Input: part model. Units: mm. Frame: model coordinates. A direction names the side the tool comes from. Give positions to 0.01 mm unless a question says otherwise; leave off trailing zeros. Loops run counter-clockwise (first coordinate to the right, second up) from the corner with the lowest first, then second, coordinate; pieces in that order, holes last. Notation, with made-up numbers: (41.5, -36) - (97.5, -36) arc R14 ccw to (97.5, -9) - close; hole circle Ø10 at (37.5, 48.25). An arc over 180 degrees is marked (long way). Answer as a JSON object with one key per item and string values. Group by question number.
(1) Mould query, pull axis Y, two halves, no side actions, for faces 1 (the flat face through (-29, -41.222, -12)), 2 (the flat face through (-27.9, -34.7, -7.2)), 3 (the cylindrical face through (-56.978, -10.627, -8.218)), 4 (the flat face through (-51, -8, 1.765)). Classes: +Y half, -Y half, draft (parallel to the pull), parting line (faces both ways), or undercut.
(2) Section query D-D (y = -31.5). Return loops of the section in (x, z).
(3) Pin query (flat end, axial travel): P1, Ø9, axis at x = -21.5, y = -17.5, coming from the -Z side; P2, Ø1.8, axis at x = -3, y = -12.5, coming from the +Z side; P3, Ø1, axis at x = -61, y = -22, coming from the +Z side. Return the tip coordinate at first contact, or that it passes through.
(4) Section query C-C (x = -14.5). Return loops of the section in (y, z).
(5) Material intervals for L1, parallel to Y at x = -25.5, z = -1; L2, parallel to X at y = -37.5, z = -5.5; L3, parallel to Z at x = -56, y = -10, sorted ascending.
(6) Section query A-A (z = -21.5). Return loops of the section in (x, y).
(7) Section query B-B (y = -24). Return loops of the section in (x, z).
(8) Access query for faces 5 (the flat face through (-32.024, -32, -7)), 6 (the flat face through (-61, -24, 1.6)), 7 (the flat face through (-30, -39.222, -20)), 8 (the cylindrical face through (-2.82, -13.2, -27.97)). Directions: +Z, -Z, +X, -X, +Y, -Y. A direction counts if a zero-diameter tool reaches every point of the face in a straight line with its end or side. Return the directions, or none.
```python
from build123d import *

# Parameters (mm, degrees)
SKETCH_2_W           = 65.2997206
SKETCH_2_H           = 34.311658624
SKETCH_2_R           = 1.00000254
SKETCH_2_R_2         = 0.922218434
SKETCH_2_R_3         = 1.5
EXTRUDE_2_DEPTH      = 4.5
SKETCH_3_R           = 1.5
CUT_EXTRUDE_2_DEPTH  = 2.5
SKETCH_5_W           = 65.2997206
SKETCH_5_H           = 34.311658624
SKETCH_5_W_2         = 61.2997206
SKETCH_5_H_2         = 30.311658624
EXTRUDE_3_DEPTH      = 15.5
EXTRUDE_3_DEPTH_BACK = 16
SKETCH_7_W           = 8.214112973
SKETCH_7_H           = 3.795011114
CUT_EXTRUDE_4_DEPTH  = 3
SKETCH_8_W           = 4
SKETCH_8_H           = 9.575559499
CUT_EXTRUDE_5_DEPTH  = 3
SKETCH_9_W           = 9.326303795
SKETCH_9_H           = 4.202278939
CUT_EXTRUDE_6_DEPTH  = 3
SKETCH_10_W          = 65.2997206
SKETCH_10_H          = 34.311658624
SKETCH_10_R          = 1
EXTRUDE_4_DEPTH      = 4


with BuildPart() as part:
    # 草图2 → 凸台-拉伸2 (new body)
    with BuildSketch(Plane(origin=(0, 0, -6), x_dir=(-1, 0, 0), z_dir=(0, 0, -1))):
        with Locations((29.273558547, -24.066548133)):
            Rectangle(SKETCH_2_W, SKETCH_2_H)
        with Locations((1.016002032, -11.24978156)):
            Circle(SKETCH_2_R, mode=Mode.SUBTRACT)
        with Locations((0.889001778, -36.83007366)):
            Circle(SKETCH_2_R, mode=Mode.SUBTRACT)
        with Locations((57.658115316, -36.64983236)):
            Circle(SKETCH_2_R, mode=Mode.SUBTRACT)
        with Locations((57.658115316, -11.24978156)):
            Circle(SKETCH_2_R_2, mode=Mode.SUBTRACT)
        with Locations((29.273558547, -32.316548133)):
            Circle(SKETCH_2_R_3, mode=Mode.SUBTRACT)
        with BuildLine():
            Line((27.785407033, -15.816548133), (27.785407033, -13.183619987))
            ThreePointArc((27.785407033, -13.183619987), (29.273558547, -11.695468472), (30.761710061, -13.183619987))
            Line((30.761710061, -13.183619987), (30.761710061, -15.816548133))
            ThreePointArc((30.761710061, -15.816548133), (29.273558547, -17.304699647), (27.785407033, -15.816548133))
        make_face(mode=Mode.SUBTRACT)
    extrude(amount=EXTRUDE_2_DEPTH)

    # 草图3 → 切除-拉伸2 (cut)
    with BuildSketch(Plane(origin=(0, 0, -6), x_dir=(-1, 0, 0), z_dir=(0, 0, -1))):
        Polygon((29.273558547, -18.991974614), (32.023558547, -17.404261373), (32.023558547, -14.920341582), (32.023558547, -14.228834893), (32.023558547, -11.744915102), (29.273558547, -10.157201862), (26.523558547, -11.744915102), (26.523558547, -14.228834893), (26.523558547, -14.920341582), (26.523558547, -17.404261373), align=None)
        with BuildLine():
            ThreePointArc((30.761710061, -15.816548133), (29.273558547, -17.304699647), (27.785407033, -15.816548133))
            Line((27.785407033, -15.816548133), (27.785407033, -13.183619987))
            ThreePointArc((27.785407033, -13.183619987), (29.273558547, -11.695468472), (30.761710061, -13.183619987))
            Line((30.761710061, -13.183619987), (30.761710061, -15.816548133))
        make_face(mode=Mode.SUBTRACT)
        Polygon((26.523558547, -30.728834893), (26.523558547, -33.904261373), (29.273558547, -35.491974614), (32.023558547, -33.904261373), (32.023558547, -30.728834893), (29.273558547, -29.141121653), align=None)
        with Locations((29.273558547, -32.316548133)):
            Circle(SKETCH_3_R, mode=Mode.SUBTRACT)
    extrude(amount=CUT_EXTRUDE_2_DEPTH, mode=Mode.SUBTRACT)

    # 草图5 → 凸台-拉伸3 (add, two sides)
    with BuildSketch(Plane(origin=(0, 0, -10.5), x_dir=(-1, 0, 0), z_dir=(0, 0, -1))) as extrude_3_sk:
        with Locations((29.273558547, -24.066548133)):
            Rectangle(SKETCH_5_W, SKETCH_5_H)
        with Locations((29.273558547, -24.066548133)):
            Rectangle(SKETCH_5_W_2, SKETCH_5_H_2, mode=Mode.SUBTRACT)
    extrude(amount=EXTRUDE_3_DEPTH)
    extrude(extrude_3_sk.sketch, amount=-EXTRUDE_3_DEPTH_BACK)

    # 草图7 → 切除-拉伸4 (cut)
    with BuildSketch(Plane(origin=(0, -6.910718821, 0), x_dir=(1, 0, 0), z_dir=(0, 1, 0))):
        with Locations((-50.955145133, -3.662545243)):
            Rectangle(SKETCH_7_W, SKETCH_7_H)
    extrude(amount=-CUT_EXTRUDE_4_DEPTH, mode=Mode.SUBTRACT)

    # 草图8 → 切除-拉伸5 (cut)
    with BuildSketch(Plane.ZY.offset(61.923418847)):
        with Locations((3.6000508, -23.483057223)):
            Rectangle(SKETCH_8_W, SKETCH_8_H)
    extrude(amount=-CUT_EXTRUDE_5_DEPTH, mode=Mode.SUBTRACT)

    # 草图9 → 切除-拉伸6 (cut)
    with BuildSketch(Plane.XZ.offset(41.222377445)):
        with Locations((-44.464129124, 3.49891133)):
            Rectangle(SKETCH_9_W, SKETCH_9_H)
    extrude(amount=-CUT_EXTRUDE_6_DEPTH, mode=Mode.SUBTRACT)

    # 草图10 → 凸台-拉伸4 (add)
    with BuildSketch(Plane(origin=(0, 0, -26), x_dir=(-1, 0, 0), z_dir=(0, 0, -1))):
        with Locations((29.273558547, -24.066548133)):
            Rectangle(SKETCH_10_W, SKETCH_10_H)
        Polygon((-1.376301753, -14.910718821), (-1.376301753, -8.910718821), (4.623698247, -8.910718821), (53.923418847, -8.910718821), (59.923418847, -8.910718821), (59.923418847, -14.910718821), (59.923418847, -33.222377445), (59.923418847, -39.222377445), (53.923418847, -39.222377445), (4.623698247, -39.222377445), (-1.376301753, -39.222377445), (-1.376301753, -33.222377445), align=None, mode=Mode.SUBTRACT)
        with BuildLine():
            Line((4.623698247, -8.910718821), (-1.376301753, -8.910718821))
            Line((-1.376301753, -8.910718821), (-1.376301753, -14.910718821))
            ThreePointArc((-1.376301753, -14.910718821), (2.866338935, -13.153359509), (4.623698247, -8.910718821))
        make_face()
        with Locations((1.016002032, -11.24978156)):
            Circle(SKETCH_10_R, mode=Mode.SUBTRACT)
        with BuildLine():
            ThreePointArc((4.623698247, -39.222377445), (2.866338935, -34.979736758), (-1.376301753, -33.222377445))
            Line((-1.376301753, -33.222377445), (-1.376301753, -39.222377445))
            Line((-1.376301753, -39.222377445), (4.623698247, -39.222377445))
        make_face()
        with Locations((1.016002032, -36.883314707)):
            Circle(SKETCH_10_R, mode=Mode.SUBTRACT)
        with BuildLine():
            Line((59.923418847, -39.222377445), (59.923418847, -33.222377445))
            ThreePointArc((59.923418847, -33.222377445), (55.68077816, -34.979736758), (53.923418847, -39.222377445))
            Line((53.923418847, -39.222377445), (59.923418847, -39.222377445))
        make_face()
        with Locations((57.658115316, -36.883314707)):
            Circle(SKETCH_10_R, mode=Mode.SUBTRACT)
        with BuildLine():
            Line((59.923418847, -8.910718821), (53.923418847, -8.910718821))
            ThreePointArc((53.923418847, -8.910718821), (55.68077816, -13.153359509), (59.923418847, -14.910718821))
            Line((59.923418847, -14.910718821), (59.923418847, -8.910718821))
        make_face()
        with Locations((57.658115316, -11.24978156)):
            Circle(SKETCH_10_R, mode=Mode.SUBTRACT)
    extrude(amount=EXTRUDE_4_DEPTH)


solid = part.part
```
Recorded:
{
 "1": {"face 1": "-Y half", "face 2": "undercut", "face 3": "undercut", "face 4": "draft"},
 "2": {"outline": "(-61.92, -30) - (-59.92, -30) - (-59.92, -10.5) - (-30.53, -10.5) - (-30.53, -8.5) - (-32.02, -8.5) - (-32.02, -6) - (-59.92, -6) - (-59.92, 5.5) - (-61.92, 5.5) - close; (-28.02, -10.5) - (1.38, -10.5) - (1.38, -30) - (3.38, -30) - (3.38, 5.5) - (1.38, 5.5) - (1.38, -6) - (-26.52, -6) - (-26.52, -8.5) - (-28.02, -8.5) - close"},
 "3": {"P1": "stops at z = -10.5", "P2": "stops at z = -6", "P3": "stops at z = 1.6"},
 "4": {"outline": "(-41.22, -30) - (-39.22, -30) - (-39.22, -10.5) - (-8.91, -10.5) - (-8.91, -30) - (-6.91, -30) - (-6.91, 5.5) - (-8.91, 5.5) - (-8.91, -6) - (-39.22, -6) - (-39.22, 5.5) - (-41.22, 5.5) - close"},
 "5": {"L1": "y = -41.22 to -39.22, -8.91 to -6.91", "L2": "x = -61.92 to -59.92, 1.38 to 3.38", "L3": "z = -30 to -26, -10.5 to -6"},
 "6": {"outline": "(-61.92, -41.22) - (3.38, -41.22) - (3.38, -6.91) - (-61.92, -6.91) - close; hole (-59.92, -39.22) - (1.38, -39.22) - (1.38, -8.91) - (-59.92, -8.91) - close"},
 "7": {"outline": "(-61.92, -30) - (-59.92, -30) - (-59.92, -10.5) - (1.38, -10.5) - (1.38, -30) - (3.38, -30) - (3.38, 5.5) - (1.38, 5.5) - (1.38, -6) - (-59.92, -6) - (-59.92, 1.6) - (-61.92, 1.6) - close"},
 "8": {"face 5": "+Z", "face 6": "+Z, -X", "face 7": "none", "face 8": "-Z"}
}
